Autodesk Inventor part; units mm, degrees
ref_plane "YZ Plane" through (0, 0, 0) normal (1, 0, 0) x (0, 1, 0)
ref_plane "XZ Plane" through (0, 0, 0) normal (0, 1, 0) x (-1, 0, 0)
ref_plane "XY Plane" through (0, 0, 0) normal (0, 0, 1) x (1, 0, 0)
sketch "Sketch1" plane through (0, 0, 0) normal (1, 0, 0) x (0, 1, 0)
  line L0 (0, 0) -> (33.909, 0)
  line L1 (59.309, 0) -> (59.309, 12.7)
  line L2 (46.609, 25.4) -> (0, 25.4)
  line L3 (0, 25.4) -> (0, 0)
  line L4 (46.609, -12.7) -> (46.609, -317.5)
  line L5 (59.309, -342.9) -> (59.309, 12.7)
  line L6 (46.609, -355.6) -> (0, -355.6)
  line L7 (0, -355.6) -> (0, -330.2)
  line L8 (0, -330.2) -> (33.909, -330.2)
  arc A0 (59.309, 12.7) -> (46.609, 25.4) centre (46.609, 12.7) ccw
  arc A1 (46.609, -12.7) -> (33.909, 0) centre (33.909, -12.7) ccw
  arc A2 (33.909, -330.2) -> (46.609, -317.5) centre (33.909, -317.5) ccw
  arc A3 (46.609, -355.6) -> (59.309, -342.9) centre (46.609, -342.9) ccw
  dimension "d5" = 25.4
  dimension "d6" = 12.7
  dimension "d7" = 12.7
  dimension "d8" = 12.7
  dimension "d9" = 381
  dimension "d10" = 25.4
  dimension "d11" = 59.309
  dimension "d15" = 59.309
extrude "Extrusion1" add sketch "Sketch1" along normal mid plane 12.7
sketch "Sketch2" plane through (-6.35, 0, 0) normal (0, -1, 0) x (1, 0, 0)
  line L0 (0, -355.6) -> (12.7, -355.6)
  line L1 (0, -330.2) -> (12.7, -330.2)
  line L2 (12.7, -355.6) -> (0, -355.6)
  line L3 (0, -355.6) -> (0, -330.2)
  line L4 (0, -330.2) -> (12.7, -330.2)
  line L5 (12.7, -330.2) -> (12.7, -355.6)
  line L6 (-3.175, -327.025) -> (15.875, -327.025)
  line L7 (15.875, -327.025) -> (15.875, -358.775)
  line L8 (-3.175, -358.775) -> (-3.175, -327.025)
  line L9 (12.7, -342.9) -> (0, -342.9)
  line L10 (-3.175, -327.025) -> (15.875, -358.775) construction
  line L11 (15.875, -327.025) -> (-3.175, -358.775) construction
  line L12 (15.875, -364.49) -> (15.875, -358.775)
  line L13 (-3.175, -358.775) -> (-3.175, -364.49)
  line L14 (-3.175, -367.03) -> (15.875, -367.03)
  line L15 (15.875, -367.03) -> (15.875, -364.49)
  line L16 (-3.175, -364.49) -> (-3.175, -367.03)
  circle A0 centre (1.27, -362.692) radius 2.54
  line L17 (6.35, -367.03) -> (6.35, -357.004) construction
  circle A1 centre (11.43, -362.692) radius 2.54
  line L18 (42.8308, -165.1) -> (-55.1073, -165.1) construction
  line L19 (0, 25.4) -> (12.7, 25.4)
  line L20 (0, 0) -> (12.7, 0)
  line L21 (12.7, 25.4) -> (0, 25.4)
  line L22 (0, 25.4) -> (0, 0)
  line L23 (0, 0) -> (12.7, 0)
  line L24 (12.7, 0) -> (12.7, 25.4)
  line L25 (-3.175, -3.175) -> (15.875, -3.175)
  line L26 (15.875, -3.175) -> (15.875, 28.575)
  line L27 (-3.175, 28.575) -> (-3.175, -3.175)
  line L28 (12.7, 12.7) -> (0, 12.7)
  line L29 (-3.175, -3.175) -> (15.875, 28.575) construction
  line L30 (15.875, -3.175) -> (-3.175, 28.575) construction
  line L31 (15.875, 34.29) -> (15.875, 28.575)
  line L32 (-3.175, 28.575) -> (-3.175, 34.29)
  line L33 (-3.175, 36.83) -> (15.875, 36.83)
  line L34 (15.875, 36.83) -> (15.875, 34.29)
  line L35 (-3.175, 34.29) -> (-3.175, 36.83)
  circle A2 centre (1.27, 32.492) radius 2.54
  line L36 (6.35, 36.83) -> (6.35, 26.804) construction
  circle A3 centre (11.43, 32.492) radius 2.54
  point P0 (0, 25.4)
  point P1 (12.7, 25.4)
  point P2 (6.35, -342.9)
  point P3 (6.35, 12.7)
  dimension "d16" = 19.05
  dimension "d17" = 31.75
  dimension "d27" = 5.08
  dimension "d28" = 4.445
extrude "Extrusion2" add sketch "Sketch2" against normal blind 8.89
fillet "Fillet1" radius 1.0583 14 edges at (0, 8.89, 36.83) (-9.525, 8.89, 16.8275) (9.525, 8.89, 16.8275) (-9.525, 8.89, -347.0275) (0, 8.89, -367.03) (9.525, 8.89, -347.0275) (6.35, 8.89, -342.9) (-6.35, 8.89, -342.9) (0, 8.89, -355.6) (0, 8.89, -330.2) (0, 8.89, 25.4) (-6.35, 8.89, 12.7) (0, 8.89, 0) (6.35, 8.89, 12.7)
properties part number "IndexRailOutSides" material "Polycarbonate, Clear"
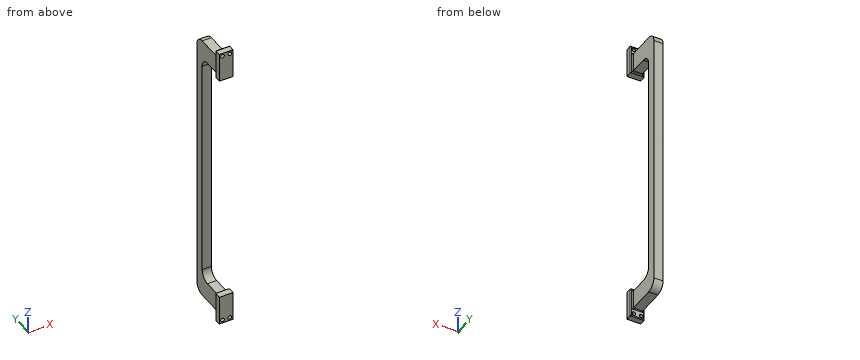
For this review, take the finished solid that the model builds, in its own axes (mm). Coordinates: 2 decimals unless noted, no trailing zeros. Loops run counter-clockwise (first coordinate to the right, second up) from the corner with the lowest first, then second, coordinate; pieces in that order, holes last.
1. Insertion check: P1, Ø5, axis at y = 49, z = -204.5, coming from the +X side; P2, Ø6.5, axis at x = 0, y = 28.5, coming from the +Z side; P3, Ø8, axis at x = -5.08, z = -362.692, coming from the +Y side. Each pin has a flat end and moves straight along its axis. Give the tip position at first contact, or say it passes through.
2. Add section C-C, the plane z = -289. Give the boundary of the cut face in (x, y).
3. For line 1 (Z direction, x = 5.08, y = 5) (3 decimals); line 2 (Y direction, x = 2.25, z = -188); line 3 (Z direction, x = -5.75, y = 41), list the stretches that pass through material, from the lowest coordinate up.
4. Add section A-A, the plane y = 17. Give the boundary of the cut face in (x, z), then the cut area to 3 significant figures.
5. Add section B-B, the plane z = -334. Give the boundary of the cut face in (x, y) (3 decimals), then the cut area to 3 significant figures.
Result:
1. P1: stops at x = 6.35
1. P2: stops at z = 25.4
1. P3: stops at y = 8.89
2. outline: (-6.35, 46.61) - (6.35, 46.61) - (6.35, 59.31) - (-6.35, 59.31) - close
3. line 1: z = -367.03 to -365.232, -360.152 to -327.025, -3.175 to 29.952, 35.032 to 36.83
3. line 2: y = 46.61 to 59.31
3. line 3: z = -355.6 to -328.04, -2.16 to 25.4
4. outline: (-6.35, -355.6) - (6.35, -355.6) - (6.35, -330.2) - (-6.35, -330.2) - close; (-6.35, 0) - (6.35, 0) - (6.35, 25.4) - (-6.35, 25.4) - close
4. area: 645 mm2
5. outline: (-9.525, 0) - (9.525, 0) - (9.525, 7.832) arc R1.058 ccw to (8.467, 8.89) - (7.408, 8.89) arc R1.058 cw to (6.35, 9.948) - (6.35, 59.309) - (-6.35, 59.309) - (-6.35, 9.948) arc R1.058 cw to (-7.408, 8.89) - (-8.467, 8.89) arc R1.058 ccw to (-9.525, 7.832) - close
5. area: 810 mm2
